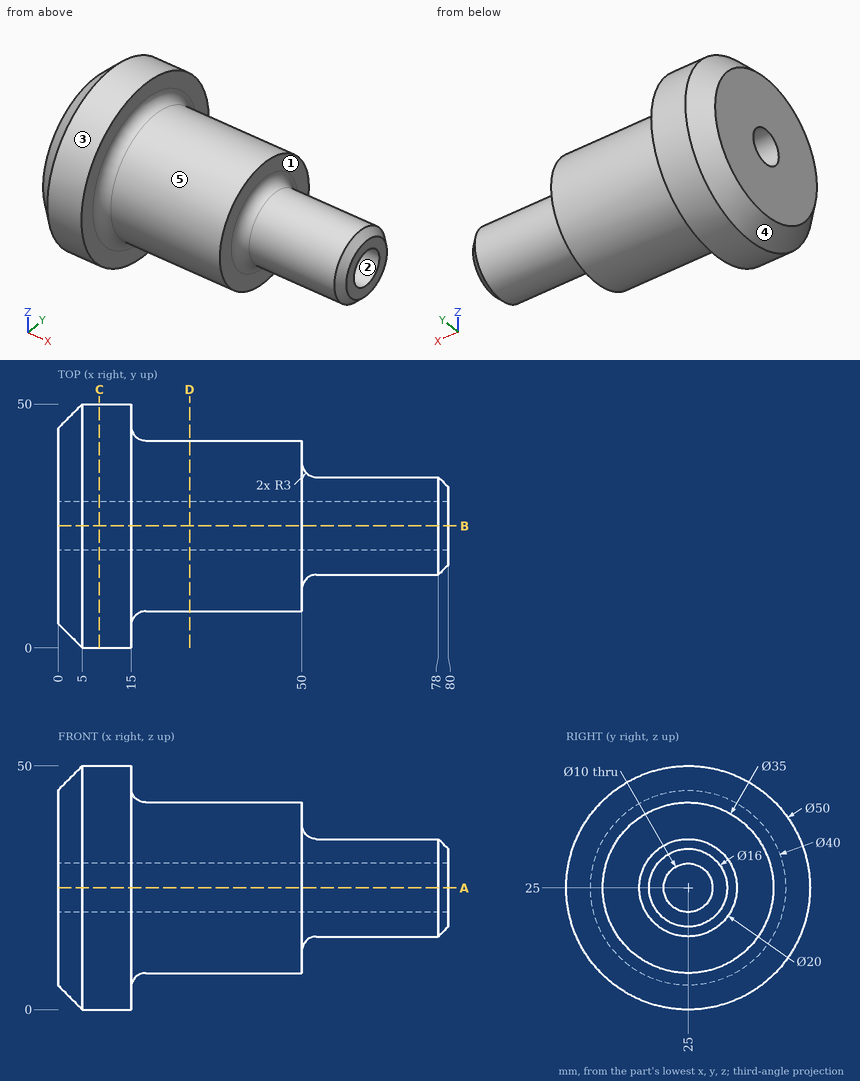
Design review of the part shown in the three views and the two pictorial views. Dimensions are in mm from the part's minimum x, y and z. A direction names the side the tool comes from. Coordinates: 2 decimals unless noted, no trailing zeros. Write each loop counter-clockwise with the first axis right and the second up, starting at its lowest first coordinate (ties: lowest second). Pieces come first, ordered by that corner, then holes.
1) Machinability: for the marked faces 4 and 5, which of the approach directions +Z, -Z, +X, -X, +Y, -Y give a long, thin tool a straight path to every point of the face, cutting with its end or side? Answer none if there is none.
2) To check wall thickness, follow probe 1 along Y at (x, z) = (62, 25); probe 2 along Y at (x, z) = (24.5, 25). State the ranges of each line that lie inside material, in increasing order.
3) We need section D-D on x = 27. State the section outline as (y, z) points.
4) Clearance check with flat-ended pins moving along their axes: pin 1 Ø10 at (x, z) = (48, 41.5) entering from +Y; pin 2 Ø3 at (y, z) = (6.5, 40) entering from +X; pin 3 Ø2 at (y, z) = (40.5, 19) entering from +X. State where each tip first meets the part, or that it passes through.
5) We need section C-C on x = 8.5. State the section outline as (y, z) points.
6) We need section A-A on z = 25. State the section outline as (x, y) points.
7) The part is to be moulded in two halves that separate along Y. For the marked faces 1, 2 and 3, say which applies: pulls with the +Y half, pulls with the -Y half, needs draft (parallel to the pull), parting line crosses it, or undercut.
Answer list:
1. face 4: -X
1. face 5: +X
2. probe 1: y = 15 to 20, 30 to 35
2. probe 2: y = 7.5 to 20, 30 to 42.5
3. outline: circle Ø35 at (25, 25); hole circle Ø10 at (25, 25)
4. pin 1: stops at y = 38.19
4. pin 2: stops at x = 15
4. pin 3: stops at x = 50
5. outline: circle Ø50 at (25, 25); hole circle Ø10 at (25, 25)
6. outline: (0, 5) - (5, 0) - (15, 0) - (15, 4.5) arc R3 cw to (18, 7.5) - (50, 7.5) - (50, 12) arc R3 cw to (53, 15) - (78, 15) - (80, 17) - (80, 20) - (0, 20) - close; (0, 30) - (80, 30) - (80, 33) - (78, 35) - (53, 35) arc R3 cw to (50, 38) - (50, 42.5) - (18, 42.5) arc R3 cw to (15, 45.5) - (15, 50) - (5, 50) - (0, 45) - close
7. face 1: needs draft
7. face 2: undercut
7. face 3: parting line crosses it
